Part model, mm, in its own coordinate system. Face numbers are marked on the shaded views. Coordinates: 2 decimals unless noted, no trailing zeros. Write each question's results on one line, items separated by ' | '.
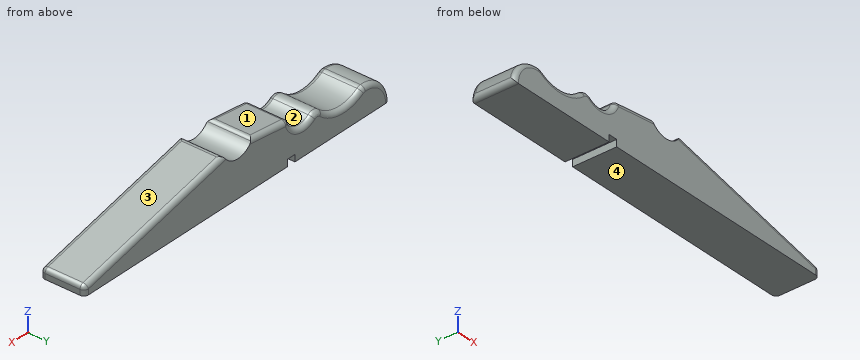
from build123d import *

# Parameters (mm, degrees)
F1_DEPTH = 9.7
F3_R     = 2
F4_R     = 1
F2_W     = 2
F2_H     = 1.5
F5_DEPTH = 9.701


with BuildPart() as f1:
    # F0 (on Front) → F1 (new body)
    with BuildSketch(Plane.XZ):
        with BuildLine():
            ThreePointArc((7, 6), (2.120195, 4.609772), (0, 0))
            Line((0, 0), (80, 0))
            Line((80, 0), (80, 2))
            Line((80, 2), (43.5, 10.3))
            ThreePointArc((43.5, 10.3), (39.75, 8), (36, 10.3))
            Line((36, 10.3), (26.5, 9.2))
            ThreePointArc((26.5, 9.2), (23.105314, 6.035142), (19, 8.2))
            ThreePointArc((19, 8.2), (13.450531, 4.642557), (7, 6))
        make_face()
    extrude(amount=F1_DEPTH)

    # F3
    f3_edges = [f1.edges().sort_by_distance(p)[0] for p in [
        (19, -4.85, 8.2),
        (7, -4.85, 6),
    ]]
    fillet(f3_edges, radius=F3_R)

    # F4
    f4_edges = [f1.edges().sort_by_distance(p)[0] for p in [
        (26.5, -4.85, 9.2),
        (36, -4.85, 10.3),
        (43.5, -4.85, 10.3),
        (80, -4.85, 2),
        (61.75, 0, 6.15),
        (61.75, -9.7, 6.15),
        (31.25, 0, 9.75),
        (31.25, -9.7, 9.75),
        (1.907739, 0, 4.418816),
        (6.432073, -4.85, 6.060708),
        (0, -4.85, 0),
        (1.907739, -9.7, 4.418816),
        (80, -9.7, 1),
        (80, 0, 1),
    ]]
    fillet(f4_edges, radius=F4_R)

    # F2 (on face) → F5 (cut, through all)
    with BuildSketch(Plane.XZ.offset(9.7)):
        with Locations((25.8, 0.75)):
            Rectangle(F2_W, F2_H)
    extrude(amount=-F5_DEPTH, mode=Mode.SUBTRACT)


solid = f1.part
(1) Two-plate mould, pull along X, no slides. Class the marked faces 1, 2, 3 and 4: released by +X, released by -X, zero draft, split by the parting line, or undercut.
Return value:
face 1: released by -X | face 2: undercut | face 3: released by +X | face 4: zero draft
(2) Wall check: line 1 (X direction, y = -8.25, z = 1.25); line 2 (Z direction, x = 12, y = -7); line 3 (Y direction, x = 45, z = 9). Give the ranges that are in metal, low to high. Write a range as from..to.
Return value:
line 1: x = 0.13..24.8, 26.8..80 | line 2: z = 0..4.5 | line 3: y = -9.7..0
(3) Flat gauge pins, fed straight in: P1, Ø1, axis at x = 25.5, y = -7, coming from the -Z side; P2, Ø1.5, axis at y = -1, z = 9, coming from the -X side; P3, Ø3, axis at y = -3.5, z = 3.5, coming from the -X side; P4, Ø3, axis at x = 9.5, y = -2, coming from the -Z side. Where does each tip first touch, or does it go through?
Return value:
P1: stops at z = 1.5 | P2: stops at x = 26.18 | P3: stops at x = 0.34 | P4: stops at z = 0
